Part model, mm, in its own coordinate system. Face numbers are marked on the shaded views. A direction names the side the tool comes from. Give positions to 0.01 mm unless a question says otherwise; leave off trailing zeros. Order: outer loops, then holes, each group sorted by start corner. A loop starts at its lowest first (then second) coordinate and runs counter-clockwise, first axis right, second up. Notation, with made-up numbers: M 38.25,-34 L 85.25,-34 A17 cw 85.25,-22 Z; hole C -29.5,20 d3. An arc over 180 degrees is marked long. Answer as a JSON object with one key per item and string values.
from build123d import *

# Parameters (mm, degrees)
SKETCH1_W           = 17.606601718
SKETCH1_H           = 38
SKETCH1_R           = 3.2
SKETCH1_R_2         = 1.65
BOSS_EXTRUDE1_DEPTH = 5
CUT_EXTRUDE4_START  = -5
SKETCH4_6_W         = 4
SKETCH4_6_H         = 25
CUT_EXTRUDE4_DEPTH  = 2
CUT_EXTRUDE1_DEPTH  = 3
CUT_EXTRUDE5_DEPTH  = 1.8


with BuildPart() as part:
    # Sketch1 → Boss-Extrude1 (new body)
    with BuildSketch(Plane.XY):
        with Locations((-0.607278146, -5.166340893)):
            Rectangle(SKETCH1_W, SKETCH1_H)
        with Locations((-2.410579005, 5.833659107)):
            Circle(SKETCH1_R, mode=Mode.SUBTRACT)
        with Locations((-5.210579005, -4.166340893)):
            Circle(SKETCH1_R_2, mode=Mode.SUBTRACT)
        with Locations((-5.210579005, -19.166340893)):
            Circle(SKETCH1_R_2, mode=Mode.SUBTRACT)
    extrude(amount=BOSS_EXTRUDE1_DEPTH)

    # Sketch4<6> → Cut-Extrude4 (cut)
    with BuildSketch(Plane.XY.offset(5).offset(CUT_EXTRUDE4_START)):
        with Locations((6.196022713, -11.666340893)):
            Rectangle(SKETCH4_6_W, SKETCH4_6_H)
    extrude(amount=CUT_EXTRUDE4_DEPTH, mode=Mode.SUBTRACT)

    # Sketch4 → Cut-Extrude1 (cut)
    with BuildSketch(Plane.XY.offset(5)):
        Polygon((-3.50739571, -1.216340893), (-6.913762299, -1.216340893), (-8.616945593, -4.166340893), (-6.913762299, -7.116340893), (-3.50739571, -7.116340893), (-1.804212416, -4.166340893), align=None)
        Polygon((-1.804212416, -19.166340893), (-3.50739571, -22.116340893), (-6.913762299, -22.116340893), (-8.616945593, -19.166340893), (-6.913762299, -16.216340893), (-3.50739571, -16.216340893), align=None)
    extrude(amount=-CUT_EXTRUDE1_DEPTH, mode=Mode.SUBTRACT)

    # Sketch4<7> → Cut-Extrude5 (cut)
    with BuildSketch(Plane.XY.offset(5)):
        with BuildLine():
            Line((8.196022713, -2.166340893), (8.196022713, -8.166340893))
            ThreePointArc((8.196022713, -8.166340893), (5.196022713, -5.166340893), (8.196022713, -2.166340893))
        make_face()
    extrude(amount=-CUT_EXTRUDE5_DEPTH, mode=Mode.SUBTRACT)


solid = part.part
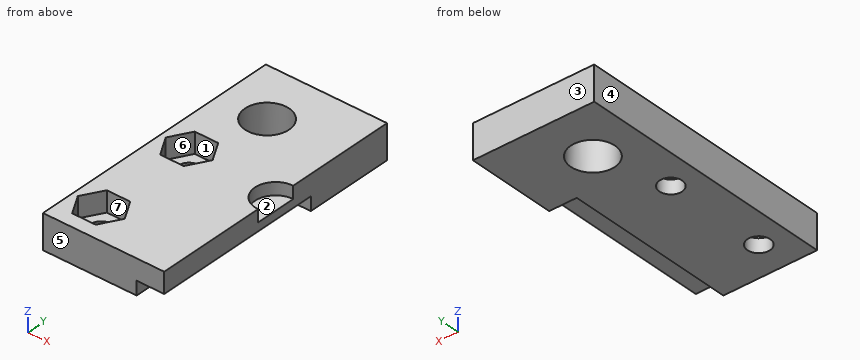
1. Probe line 1 along Y through (x, z) = (-5, 0.65); line 2 along X through (y, z) = (3, 4.6); line 3 along Y through (x, z) = (-3, 1.6). List the from-to ranges inside material, lowest first.
Worked answers:
{"line 1": "y = -24.17 to -20.8, -17.53 to -5.8, -2.53 to 3.95, 7.71 to 13.83", "line 2": "x = -9.41 to -3.9, -0.92 to 8.2", "line 3": "y = -24.17 to 2.69, 8.98 to 13.83"}
2. Cut at C-C on y = -15.5. Give the cut face in (x, z).
Worked answers:
{"outline": "M -9.41,0 L 4.2,0 L 4.2,2 L 8.2,2 L 8.2,5 L -9.41,5 Z"}
3. Cut at B-B on z = 3.95. Give the cut face in (x, y).
Worked answers:
{"outline": "M -9.41,-24.17 L 8.2,-24.17 L 8.2,-8.17 A3 cw 8.2,-2.17 L 8.2,13.83 L -9.41,13.83 Z; hole M -8.62,-19.17 L -6.91,-22.12 L -3.51,-22.12 L -1.8,-19.17 L -3.51,-16.22 L -6.91,-16.22 Z; hole M -8.62,-4.17 L -6.91,-7.12 L -3.51,-7.12 L -1.8,-4.17 L -3.51,-1.22 L -6.91,-1.22 Z; hole C -2.41,5.83 d6.4"}
4. Which spindle directions (+Z, -Z, +X, -X, +Y, -Y) get a long thin tool onto all of the face, cutting with end or side? Do the marked faces 1, 2 and 3. Say none if no direction does.
Worked answers:
{"face 1": "+Z", "face 2": "+Z, +X", "face 3": "+Z, -Z, +X, -X, +Y"}
5. Cut at A-A on x = -5. Give the cut face in (y, z).
Worked answers:
{"outline": "M -24.17,0 L -20.8,0 L -20.8,2 L -22.12,2 L -22.12,5 L -24.17,5 Z; M -17.53,0 L -5.8,0 L -5.8,2 L -7.12,2 L -7.12,5 L -16.22,5 L -16.22,2 L -17.53,2 Z; M -2.53,0 L 3.95,0 L 3.95,5 L -1.22,5 L -1.22,2 L -2.53,2 Z; M 7.71,0 L 13.83,0 L 13.83,5 L 7.71,5 Z"}
6. Cut at D-D on y = 3.5. Give the cut face in (x, z), plus the area to 3 significant figures.
Worked answers:
{"outline": "M -9.41,0 L -4.6,0 L -4.6,5 L -9.41,5 Z; M -0.22,0 L 8.2,0 L 8.2,5 L -0.22,5 Z", "area": "66.1 mm^2"}
7. Pin check, flat tips, straight feed: P1, Ø1.8, axis at x = -6, y = -18, coming from the +Z side; P2, Ø1.2, axis at x = 6, y = -6, coming from the -Z side; P3, Ø3.5, axis at x = 7.5, y = -6, coming from the +Z side. Stop position of each tip, or through.
Worked answers:
{"P1": "stops at z = 2", "P2": "stops at z = 2", "P3": "stops at z = 3.2"}
8. Two-plate mould, pull along X, no slides. Class the marked faces 4, 5, 6 and 7: +X half, -X half, draft (parallel to the pull), parting line (faces both ways), or undercut.
Worked answers:
{"face 4": "-X half", "face 5": "draft", "face 6": "undercut", "face 7": "undercut"}
